Work out the finished part from the listing and answer in its coordinate system (mm). Round coordinates to 2 decimals unless told otherwise and drop trailing zeros. Loops run counter-clockwise (first coordinate to the right, second up) from the corner with the lowest first, then second, coordinate; pieces in that order, holes last. Notation, with made-up numbers: (-29.75, 74.25) - (1.25, 74.25) arc R21 ccw to (1.25, 81.25) - close; hole circle Ø6 at (59, -12). An arc over 180 degrees is marked (long way). Return JSON: item names as keys, results as strings.
from build123d import *

# Parameters (mm, degrees)
SKETCH_W        = 12.7
SKETCH_H        = 88.9
PAD_DEPTH       = 717.5
SKETCH001_W     = 6.35
SKETCH001_H     = 12.7
POCKET_DEPTH    = 717.501
SKETCH002_W     = 6.35
SKETCH002_H     = 6.35
POCKET001_DEPTH = 88.901
SKETCH003_R     = 3
HOLE_DEPTH      = 12.701


with BuildPart() as part:
    # Sketch → Pad (new body)
    with BuildSketch(Plane.YZ):
        with Locations((6.35, 44.45)):
            Rectangle(SKETCH_W, SKETCH_H)
    extrude(amount=PAD_DEPTH)

    # Sketch001 (on Face6 of Pad) → Pocket (cut, through all)
    with BuildSketch(Plane.YZ.offset(717.5)):
        with Locations((9.525, 12.7)):
            Rectangle(SKETCH001_W, SKETCH001_H)
    extrude(amount=-POCKET_DEPTH, mode=Mode.SUBTRACT)

    # Sketch002 (on Face6 of Pocket) → Pocket001 (cut, through all)
    with BuildSketch(Plane(origin=(0, 0, 88.9), x_dir=(0, -1, 0), z_dir=(0, 0, 1))):
        with Locations((-9.525, 714.325)):
            Rectangle(SKETCH002_W, SKETCH002_H)
        with Locations((-9.525, 3.175)):
            Rectangle(SKETCH002_W, SKETCH002_H)
    extrude(amount=-POCKET001_DEPTH, mode=Mode.SUBTRACT)

    # Sketch003 (on Face9 of Pocket001) → Hole (cut, through all)
    with BuildSketch(Plane(origin=(0, 0, 0), x_dir=(0, 0, -1), z_dir=(0, -1, 0))):
        with Locations((-44.45, 310.75)):
            Circle(SKETCH003_R)
        with Locations((-44.45, 406.75)):
            Circle(SKETCH003_R)
    extrude(amount=-HOLE_DEPTH, mode=Mode.SUBTRACT)


solid = part.part
1) Section B-B (x = 639) is taken. Give the vertices of the cut face in (y, z), and give its area (3 significant figures).
Verdict:
{"outline": "(0, 0) - (12.7, 0) - (12.7, 6.35) - (6.35, 6.35) - (6.35, 19.05) - (12.7, 19.05) - (12.7, 88.9) - (0, 88.9) - close", "area": "1,050 mm2"}
2) Find the intervals of material crossed by L1, parallel to X at y = 9, z = 45; L2, parallel to Z at x = 310.75, y = 8.25; L3, parallel to Z at x = 370, y = 8, in increasing order.
Verdict:
{"L1": "x = 6.35 to 307.8, 313.7 to 403.8, 409.7 to 711.15", "L2": "z = 0 to 6.35, 19.05 to 41.45, 47.45 to 88.9", "L3": "z = 0 to 6.35, 19.05 to 88.9"}
3) Determine the mould class of faces 1 (the flat face through (354, 6, 0)), 2 (the flat face through (354, 0, 44)), 3 (the flat face through (357, 6.35, 15)), 4 (the flat face through (354, 6, 88.9)) for opening direction Z: pulls with the +Z half, pulls with the -Z half, needs draft (parallel to the pull), parting line crosses it, or undercut.
Verdict:
{"face 1": "pulls with the -Z half", "face 2": "needs draft", "face 3": "undercut", "face 4": "pulls with the +Z half"}
4) Section A-A (y = 10) is taken. Give the vertices of the cut face in (x, z).
Verdict:
{"outline": "(6.35, 0) - (711.15, 0) - (711.15, 6.35) - (6.35, 6.35) - close; (6.35, 19.05) - (711.15, 19.05) - (711.15, 88.9) - (6.35, 88.9) - close; hole circle Ø6 at (310.75, 44.45); hole circle Ø6 at (406.75, 44.45)"}
5) Flat-ended cylindrical pins translate along their axes: pin 1 (5 mm diameter, centred on y = 9, z = 3, fed in from +X); pin 2 (5 mm diameter, centred on y = 9.5, z = 42, fed in from -X). Find the tip coordinate at first contact, or state that the pin passes through.
Verdict:
{"pin 1": "stops at x = 711.15", "pin 2": "stops at x = 6.35"}
